Can you work these out from the model? Positions are in its coordinate system, mm. A direction names the side the tool comes from. Give positions to 0.01 mm unless a question says otherwise; leave off trailing zeros. Write each loop counter-clockwise with the first axis right and the second up, starting at its lowest first coordinate (ties: lowest second). Pieces come first, ordered by that corner, then holes. Notation, with made-up numbers: (5, 14.25) -> (33, 14.25) arc R26 cw to (33, 53.25) -> close; hole circle Ø5 at (81.25, -27.5). An arc over 180 degrees is marked (long way). Answer as CSV lines item,"result". Start each with the question number.
1. I'm going to push flat-ended pins straight in: P1, Ø1.8, axis at x = 62, z = 4, coming from the +Y side; P2, Ø5, axis at x = 45, y = 0.5, coming from the +Z side; P3, Ø7, axis at x = -43.5, y = 41, coming from the +Z side (3 decimals); P4, Ø4, axis at x = 62.82, y = 32.54, coming from the -Z side. Where does each tip first touch, or does it pass through?
2. If we section it at B-B on x = -15.5: Write out the boundary of the cut face in (y, z).
3. On a 3-axis mill with a long thin cutter (end or side, diameter ignored), from which of +Z, -Z, +X, -X, +Y, -Y can I reach the whole of each face in a straight line? I mean faces 1 (the face through (46.5, 39.4, 21.875)), 2 (the face through (69.86, 39.626, 3.042)), 3 (the face through (-47, 41, 17.43)). Say none if no direction works.
4. If we section it at A-A on z = 9: Count the separate pieces of the cut face and the enclosed holes in it, plus the area to 3 significant figures.
5. If we mould it in two halves opening along X, with no side actions, what happens to faces 4 (the face through (55.74, 23.7, 3.04)), 5 (the face through (63, 24.606, 3)), 6 (the face through (-39.194, 43.567, 19.621))? For each: pulls with the +X half, pulls with the -X half, needs draft (parallel to the pull), parting line crosses it, or undercut.
6. If we section it at D-D on y = -22: Write out the boundary of the cut face in (x, z).
7. If we section it at C-C on z = 30.5: Write out the boundary of the cut face in (x, y), plus the area to 3 significant figures.
8. I need wall thicknesses on line 1 (Y direction, x = -46, z = 21); line 2 (X direction, y = 41, z = 11); line 3 (X direction, y = -43, z = 8). Which ranges of each line are inside material? Lowest first, please. Write a range as [from, to].
```python
from build123d import *

# Parameters (mm, degrees)
SKETCH1_W            = 104.775
SKETCH1_H            = 106.3625
BOSS_EXTRUDE1_DEPTH  = 6
BOSS_EXTRUDE2_DEPTH  = 38.1
SKETCH3_R            = 5
SKETCH3_R_2          = 3.025
BOSS_EXTRUDE3_DEPTH  = 15.875
SKETCH4_R            = 7
SKETCH4_R_2          = 3.025
BOSS_EXTRUDE4_DEPTH  = 11.43
BOSS_EXTRUDE5_DEPTH  = 6
M4_CLEARANCE_HOLE1_D = 4.5
FILLET2_R            = 3
FILLET3_R            = 1


with BuildPart() as part:
    # Sketch1 → Boss-Extrude1 (new body)
    with BuildSketch(Plane.XY):
        Rectangle(SKETCH1_W, SKETCH1_H)
    extrude(amount=BOSS_EXTRUDE1_DEPTH)

    # Sketch2 → Boss-Extrude2 (add)
    with BuildSketch(Plane.XY):
        Polygon((-52.3875, -53.18125), (-52.3875, -55.68125), (54.8875, -55.68125), (54.8875, 53.18125), (52.3875, 53.18125), (52.3875, -53.18125), align=None)
    extrude(amount=BOSS_EXTRUDE2_DEPTH)

    # Sketch3 → Boss-Extrude3 (add)
    with BuildSketch(Plane.XY.offset(6)):
        with Locations((43.208, 39.35095)):
            Circle(SKETCH3_R)
        with Locations((43.208, 39.35095)):
            Circle(SKETCH3_R_2, mode=Mode.SUBTRACT)
        with Locations((-41.882, 39.35095)):
            Circle(SKETCH3_R)
        with Locations((-41.882, 39.35095)):
            Circle(SKETCH3_R_2, mode=Mode.SUBTRACT)
        with Locations((-41.882, -47.00905)):
            Circle(SKETCH3_R)
        with Locations((-41.882, -47.00905)):
            Circle(SKETCH3_R_2, mode=Mode.SUBTRACT)
        with Locations((43.208, -47.00905)):
            Circle(SKETCH3_R)
        with Locations((43.208, -47.00905)):
            Circle(SKETCH3_R_2, mode=Mode.SUBTRACT)
    extrude(amount=BOSS_EXTRUDE3_DEPTH)

    # Sketch4 → Boss-Extrude4 (add)
    with BuildSketch(Plane.XY.offset(6)):
        with Locations((43.208, 39.35095)):
            Circle(SKETCH4_R)
        with Locations((43.208, 39.35095)):
            Circle(SKETCH4_R_2, mode=Mode.SUBTRACT)
        with Locations((-41.882, 39.35095)):
            Circle(SKETCH4_R)
        with Locations((-41.882, 39.35095)):
            Circle(SKETCH4_R_2, mode=Mode.SUBTRACT)
        with Locations((-41.882, -47.00905)):
            Circle(SKETCH4_R)
        with Locations((-41.882, -47.00905)):
            Circle(SKETCH4_R_2, mode=Mode.SUBTRACT)
        with Locations((43.208, -47.00905)):
            Circle(SKETCH4_R)
        with Locations((43.208, -47.00905)):
            Circle(SKETCH4_R_2, mode=Mode.SUBTRACT)
    extrude(amount=BOSS_EXTRUDE4_DEPTH)

    # Sketch6 → Boss-Extrude5 (add)
    with BuildSketch(Plane.XY):
        Polygon((-52.3875, -55.68125), (-52.3875, -39.80625), (-68.2625, -39.80625), align=None)
        Polygon((-68.2625, -55.68125), (-68.2625, -39.80625), (-52.3875, -55.68125), align=None)
        Polygon((54.8875, 24.60625), (70.7625, 40.48125), (70.7625, 24.60625), align=None)
        Polygon((54.8875, 40.48125), (54.8875, 24.60625), (70.7625, 40.48125), align=None)
    extrude(amount=BOSS_EXTRUDE5_DEPTH)

    # M4 Clearance Hole1 (through all)
    with Locations(Plane.XY.offset(6)):
        with Locations((62.825, 32.54375), (-60.325, -47.74375)):
            Hole(M4_CLEARANCE_HOLE1_D / 2)

    # Fillet2
    fillet2_edges = [part.edges().sort_by_distance(p)[0] for p in [
        (-52.3875, -39.80625, 3),
        (-68.2625, -39.80625, 3),
        (-68.2625, -55.68125, 3),
        (70.7625, 24.60625, 3),
        (70.7625, 40.48125, 3),
        (54.8875, 40.48125, 3),
        (54.8875, 24.60625, 3),
        (-52.3875, 53.18125, 3),
    ]]
    fillet(fillet2_edges, radius=FILLET2_R)

    # Fillet3
    fillet3_edges = [part.edges().sort_by_distance(p)[0] for p in [
        (-52.3875, -53.18125, 22.05),
        (-52.3875, -55.68125, 22.05),
        (54.8875, -55.68125, 19.05),
        (0, -53.18125, 38.1),
        (-52.3875, -54.43125, 38.1),
        (1.25, -55.68125, 38.1),
        (54.8875, -1.25, 38.1),
        (53.6375, 53.18125, 38.1),
        (52.3875, 0, 38.1),
    ]]
    fillet(fillet3_edges, radius=FILLET3_R)


solid = part.part
```
Computed values:
1,P1,"stops at y = 40.48"
1,P2,"stops at z = 6"
1,P3,"stops at z = 21.875"
1,P4,"passes through"
2,outline,"(-55.68, 0) -> (53.18, 0) -> (53.18, 6) -> (-53.18, 6) -> (-53.18, 37.1) arc R1 ccw to (-54.18, 38.1) -> (-54.68, 38.1) arc R1 ccw to (-55.68, 37.1) -> close"
3,face 1,"+Z, -X, +Y"
3,face 2,"+Z, -Z, +X, +Y"
3,face 3,"+Z"
4,separate pieces,"3"
4,enclosed holes,"4"
4,area,"1,030 mm2"
5,face 4,"pulls with the +X half"
5,face 5,"needs draft"
5,face 6,"undercut"
6,outline,"(-52.39, 0) -> (54.89, 0) -> (54.89, 37.1) arc R1 ccw to (53.89, 38.1) -> (53.39, 38.1) arc R1 ccw to (52.39, 37.1) -> (52.39, 6) -> (-52.39, 6) -> close"
7,outline,"(-52.39, -54.68) arc R1 ccw to (-51.39, -55.68) -> (53.89, -55.68) arc R1 ccw to (54.89, -54.68) -> (54.89, 53.18) -> (52.39, 53.18) -> (52.39, -53.18) -> (-51.39, -53.18) arc R1 ccw to (-52.39, -54.18) -> close"
7,area,"533 mm2"
8,line 1,"y = [-55.68, -53.18], [-49.84, -44.17], [36.52, 42.19]"
8,line 2,"x = [-48.68, -44.42], [-39.35, -35.08], [36.41, 40.67], [45.74, 50.01], [52.39, 54.89]"
8,line 3,"x = [-47.62, -36.14], [37.47, 48.95], [52.39, 54.89]"
